```python
from build123d import *

# Parameters (mm, degrees)
F0_R         = 26.25
F1_DEPTH     = 7
F2_R         = 13.25
F3_DEPTH     = 25.4
F4_R         = 10.16
F4_R_2       = 9.6723514766
F5_DEPTH     = 25.4
F6_T2_ANGLE  = 101.8963155292
F6_T4_ANGLE  = 100.8121389037
F6_T6_ANGLE  = 100.8121389037
F6_T8_ANGLE  = 100.8121389037
F6_T10_ANGLE = 100.8121389037
F6_T12_ANGLE = 101.8963155292
F6_T14_ANGLE = 101.8963155292
F6_T16_ANGLE = 101.8963155292


# Not quite as in the source:
# - a fillet or chamfer that OpenCascade refuses, or shapes differently, is made with other operations: its cross-section is extruded or revolved along the edge and cut away or added


with BuildPart() as f1:
    # F0 (on Top) → F1 (new body)
    with BuildSketch(Plane.XY):
        Circle(F0_R)
    extrude(amount=F1_DEPTH)

    # F2 (on face) → F3 (cut)
    with BuildSketch(Plane.XY.offset(7)):
        Circle(F2_R)
    extrude(amount=-F3_DEPTH, mode=Mode.SUBTRACT)

    # F4 (on face) → F5 (cut)
    with BuildSketch(Plane.XY.offset(7)):
        with Locations((0, -26.25)):
            Circle(F4_R)
        with Locations((-26.25, 0)):
            Circle(F4_R)
        with Locations((0, 26.25)):
            Circle(F4_R)
        with Locations((26.25, 0)):
            Circle(F4_R_2)
    extrude(amount=-F5_DEPTH, mode=Mode.SUBTRACT)

    # F6: fillet of radius 5.08 on 8 edges, made by hand

    # F6_s1 → F6_t2 (revolve, cut)
    with BuildSketch(Plane(origin=(0, 0, 0), x_dir=(0, 0, 1), z_dir=(-0.995551765, 0.0942161515, 0))):
        with BuildLine():
            ThreePointArc((5.08, -26.25), (1.4878975516, -24.7621024484), (0, -21.17))
            Line((0, -21.17), (0, -26.25))
            Line((0, -26.25), (5.08, -26.25))
        make_face()
    revolve(axis=Axis((0, 0, 0), (0, 0, 1)), revolution_arc=F6_T2_ANGLE, mode=Mode.SUBTRACT)

    # F6_s3 → F6_t4 (revolve, cut)
    with BuildSketch(Plane(origin=(0, 0, 0), x_dir=(0, 0, 1), z_dir=(0.0942137746, 0.9955519899, 0))):
        with BuildLine():
            ThreePointArc((5.08, -26.25), (1.4878975516, -24.7621024484), (0, -21.17))
            Line((0, -21.17), (0, -26.25))
            Line((0, -26.25), (5.08, -26.25))
        make_face()
    revolve(axis=Axis((0, 0, 0), (0, 0, 1)), revolution_arc=F6_T4_ANGLE, mode=Mode.SUBTRACT)

    # F6_s5 → F6_t6 (revolve, cut)
    with BuildSketch(Plane(origin=(0, 0, 0), x_dir=(0, 0, 1), z_dir=(0.9955519899, -0.0942137746, 0))):
        with BuildLine():
            ThreePointArc((5.08, -26.25), (1.4878975516, -24.7621024484), (0, -21.17))
            Line((0, -21.17), (0, -26.25))
            Line((0, -26.25), (5.08, -26.25))
        make_face()
    revolve(axis=Axis((0, 0, 0), (0, 0, 1)), revolution_arc=F6_T6_ANGLE, mode=Mode.SUBTRACT)

    # F6_s7 → F6_t8 (revolve, cut)
    with BuildSketch(Plane(origin=(0, 0, 0), x_dir=(0, 0, 1), z_dir=(0.9955519899, -0.0942137746, 0))):
        with BuildLine():
            ThreePointArc((1.92, -26.25), (5.5121024484, -24.7621024484), (7, -21.17))
            Line((7, -21.17), (7, -26.25))
            Line((7, -26.25), (1.92, -26.25))
        make_face()
    revolve(axis=Axis((0, 0, 7), (0, 0, 1)), revolution_arc=F6_T8_ANGLE, mode=Mode.SUBTRACT)

    # F6_s9 → F6_t10 (revolve, cut)
    with BuildSketch(Plane(origin=(0, 0, 0), x_dir=(0, 0, 1), z_dir=(0.0942137746, 0.9955519899, 0))):
        with BuildLine():
            ThreePointArc((1.92, -26.25), (5.5121024484, -24.7621024484), (7, -21.17))
            Line((7, -21.17), (7, -26.25))
            Line((7, -26.25), (1.92, -26.25))
        make_face()
    revolve(axis=Axis((0, 0, 7), (0, 0, 1)), revolution_arc=F6_T10_ANGLE, mode=Mode.SUBTRACT)

    # F6_s11 → F6_t12 (revolve, cut)
    with BuildSketch(Plane(origin=(0, 0, 0), x_dir=(0, 0, 1), z_dir=(-0.995551765, 0.0942161515, 0))):
        with BuildLine():
            ThreePointArc((1.92, -26.25), (5.5121024484, -24.7621024484), (7, -21.17))
            Line((7, -21.17), (7, -26.25))
            Line((7, -26.25), (1.92, -26.25))
        make_face()
    revolve(axis=Axis((0, 0, 7), (0, 0, 1)), revolution_arc=F6_T12_ANGLE, mode=Mode.SUBTRACT)

    # F6_s13 → F6_t14 (revolve, cut)
    with BuildSketch(Plane(origin=(0, 0, 0), x_dir=(0, 0, 1), z_dir=(-0.1130316961, -0.9935913826, 0))):
        with BuildLine():
            ThreePointArc((1.92, -26.25), (5.5121024484, -24.7621024484), (7, -21.17))
            Line((7, -21.17), (7, -26.25))
            Line((7, -26.25), (1.92, -26.25))
        make_face()
    revolve(axis=Axis((0, 0, 7), (0, 0, 1)), revolution_arc=F6_T14_ANGLE, mode=Mode.SUBTRACT)

    # F6_s15 → F6_t16 (revolve, cut)
    with BuildSketch(Plane(origin=(0, 0, 0), x_dir=(0, 0, 1), z_dir=(-0.1130316961, -0.9935913826, 0))):
        with BuildLine():
            ThreePointArc((5.08, -26.25), (1.4878975516, -24.7621024484), (0, -21.17))
            Line((0, -21.17), (0, -26.25))
            Line((0, -26.25), (5.08, -26.25))
        make_face()
    revolve(axis=Axis((0, 0, 0), (0, 0, 1)), revolution_arc=F6_T16_ANGLE, mode=Mode.SUBTRACT)


solid = f1.part
```
Check sheet for the modelled part. Datum: model origin and axes. Units: mm. Round coordinates to 2 decimals unless told otherwise and drop trailing zeros. Order: outer loops, then holes, each group sorted by start corner. A loop starts at its lowest first (then second) coordinate and runs counter-clockwise, first axis right, second up.
1) Section check B-B (y = 0). Record the boundary of the cut face in (x, z).
2) Go/stop test with flat-tipped pins: pin 1 Ø8 at (x, y) = (0.5, 10.5) entering from -Z; pin 2 Ø16 at (x, y) = (0, 0) entering from +Z; pin 3 Ø1 at (y, z) = (19, 6) entering from -X; pin 4 Ø1 at (y, z) = (-17.5, 3) entering from -X. Record where each tip stops, or that it passes through.
3) Section check C-C (z = 5.5). Record the boundary of the cut face in (x, y).
4) Section check A-A (x = 0). Record the boundary of the cut face in (y, z).
5) Scan lines: line 1 (X direction, y = 8.5, z = 5.5); line 2 (Y direction, x = -19.5, z = 5.5); line 3 (X direction, y = 19, z = 1.25). Record each from-to range of solid material in increasing order.
6) Section check D-D (z = 1.25). Record the boundary of the cut face in (x, y), and give its area (3 significant figures).
7) Mould release check, pull along X, two halves, no side actions. Record for faces 1 (the cylindrical face through (-16.09, -0.19, 3.55)), 2 (the flat face through (-0.2, 13.4, 0)), 3 (the cylindrical face through (16.58, 0.18, 3.55)), 4 (the cylindrical face through (-0.19, 16.09, 3.55)): +X half, -X half, draft (parallel to the pull), parting line (faces both ways), or undercut.
Result:
1. outline: (-16.09, 0) - (-13.25, 0) - (-13.25, 7) - (-16.09, 7) - close; (13.25, 0) - (16.58, 0) - (16.58, 7) - (13.25, 7) - close
2. pin 1: stops at z = 0
2. pin 2: passes through
2. pin 3: stops at x = -16.09
2. pin 4: stops at x = -19.49
3. outline: (-22.85, -9.57) arc R24.77 ccw to (-9.57, -22.85) arc R10.16 cw to (9.57, -22.85) arc R24.77 ccw to (23.03, -9.12) arc R9.67 cw to (23.03, 9.12) arc R24.77 ccw to (9.57, 22.85) arc R10.16 cw to (-9.57, 22.85) arc R24.77 ccw to (-22.85, 9.57) arc R10.16 cw to start; hole circle Ø26.5 at (0, 0)
4. outline: (-16.09, 0) - (-13.25, 0) - (-13.25, 7) - (-16.09, 7) - close; (13.25, 0) - (16.09, 0) - (16.09, 7) - (13.25, 7) - close
5. line 1: x = -20.68 to -10.16, 10.16 to 21.63
5. line 2: y = -15.28 to -7.59, 7.59 to 15.28
5. line 3: x = -15.48 to -7.12, 7.12 to 15.48
6. outline: (-22.6, -9.48) arc R24.51 ccw to (-9.48, -22.6) arc R10.16 cw to (9.48, -22.6) arc R24.51 ccw to (22.78, -9.03) arc R9.67 cw to (22.78, 9.03) arc R24.51 ccw to (9.48, 22.6) arc R10.16 cw to (-9.48, 22.6) arc R24.51 ccw to (-22.6, 9.48) arc R10.16 cw to start; hole circle Ø26.5 at (0, 0)
6. area: 891 mm2
7. face 1: -X half
7. face 2: draft
7. face 3: +X half
7. face 4: undercut
